Verification items for the finished model (mm, model axes). Coordinates: 2 decimals unless noted, no trailing zeros. Order: outer loops, then holes, each group sorted by start corner. A loop starts at its lowest first (then second) coordinate and runs counter-clockwise, first axis right, second up. Notation, with made-up numbers: (60.25, 44.5) -> (100.25, 44.5) arc R15 cw to (100.25, 52.5) -> close; hole circle Ø11 at (26.5, 33). An arc over 180 degrees is marked (long way). Answer as CSV lines item,"result".
Autodesk Inventor part; units mm, degrees
ref_plane "YZ Plane" through (0, 0, 0) normal (1, 0, 0) x (0, 1, 0)
ref_plane "XZ Plane" through (0, 0, 0) normal (0, 1, 0) x (-1, 0, 0)
ref_plane "XY Plane" through (0, 0, 0) normal (0, 0, 1) x (1, 0, 0)
sketch "Sketch1" plane through (0, 0, 0) normal (1, 0, 0) x (0, 1, 0)
  circle A0 centre (0, 0) radius 45
  circle A1 centre (0, 0) radius 7.5
  dimension "d0" = 90
  dimension "d1" = 15
extrude "Extrusion1" add sketch "Sketch1" along normal blind 5
sketch "Sketch2" plane through (5, 0, 0) normal (1, 0, 0) x (0, 0, -1)
  line L0 (0, 0) -> (-35, 0)
  circle A0 centre (-35, 0) radius 7.5
  dimension "d6" = 35
  dimension "d7" = 15
extrude "Extrusion2" cut sketch "Sketch2" against normal blind 5
sketch "Sketch3" plane through (5, 0, 0) normal (1, 0, 0) x (0, 0, -1)
  point P0 (0, 0)
sketch "Sketch4" plane through (0, 0, 0) normal (-1, 0, 0) x (0, 0, 1)
  circle A0 centre (0, 0) radius 7.5
  circle A1 centre (0, 0) radius 7.5
extrude "Extrusion3" add sketch "Sketch4" against normal blind 5
sketch "Sketch5" plane through (5, 0, 0) normal (1, 0, 0) x (0, 0, -1)
  point P0 (0, 0)
sketch "Sketch6" plane through (0, 0, 0) normal (-1, 0, 0) x (0, 0, 1)
  circle A0 centre (0, 0) radius 7.25
  dimension "d12" = 14.5
extrude "Extrusion4" add sketch "Sketch6" along normal blind 50
equation "\"BendRadius\" = Thickness"
equation "\"BendReliefWidth\" = Thickness"
equation "\"BendReliefDepth\" = 0.5 * Thickness"
equation "\"CornerReliefSize\" = 4 * Thickness"
equation "\"MinimumRemnant\" = 2 * Thickness"
equation "\"TransitionRadius\" = BendRadius"
equation "\"JacobiRadiusSize\" = BendRadius"
equation "\"GapSize\" = Thickness"
properties part number "Manivela"
Item 1: Section check D-D, the plane x = -15. Record the boundary of the cut face in (y, z), plus the area to 3 significant figures.
Answer list:
outline,"circle Ø14.5 at (0, 0)"
area,"165 mm2"
Item 2: Section check A-A, the plane y = 0. Record the boundary of the cut face in (x, z), plus the area to 3 significant figures.
Answer list:
outline,"(-50, -7.25) -> (0, -7.25) -> (0, -45) -> (5, -45) -> (5, 27.5) -> (0, 27.5) -> (0, 7.25) -> (-50, 7.25) -> close; (0, 42.5) -> (5, 42.5) -> (5, 45) -> (0, 45) -> close"
area,"1,100 mm2"
Item 3: Depth check by flat-ended pin: pin 1 Ø12 at (y, z) = (30.5, -22.5) entering from -X; pin 2 Ø6 at (x, z) = (-41.5, -8) entering from +Y; pin 3 Ø8 at (x, y) = (-36, 13.5) entering from -Z. Enter the tip coordinate at first touch or a pass-through.
Answer list:
pin 1,"x = 0"
pin 2,"y = 5.25"
pin 3,"through"
Item 4: Thickness scan on line 1 (X direction, y = -5, z = -19.5); line 2 (Y direction, x = 2, z = 35); line 3 (Y direction, x = -17, z = -4.5). Record the ranges inside material, lowest first.
Answer list:
line 1,"0 to 5"
line 2,"-28.28 to -7.5, 7.5 to 28.28"
line 3,"-5.68 to 5.68"
Item 5: Section check C-C, the plane z = 0. Record the boundary of the cut face in (x, y).
Answer list:
outline,"(-50, -7.25) -> (0, -7.25) -> (0, -45) -> (5, -45) -> (5, 45) -> (0, 45) -> (0, 7.25) -> (-50, 7.25) -> close"
Item 6: Release check for a two-part mould opening along Z. For faces 1 (the cylindrical face through (2.535, 0.33, 42.493)), 2 (the cylindrical face through (-24.65, 6.43, 3.35)), 3 (the flat face through (5, -1, 1)) record: +Z half, -Z half, draft (parallel to the pull), parting line (faces both ways), or undercut.
Answer list:
face 1,"undercut"
face 2,"parting line"
face 3,"draft"
Item 7: Section check B-B, the plane z = 36.5. Record the boundary of the cut face in (x, y).
Answer list:
outline,"(0, -26.32) -> (5, -26.32) -> (5, -7.35) -> (0, -7.35) -> close; (0, 7.35) -> (5, 7.35) -> (5, 26.32) -> (0, 26.32) -> close"
